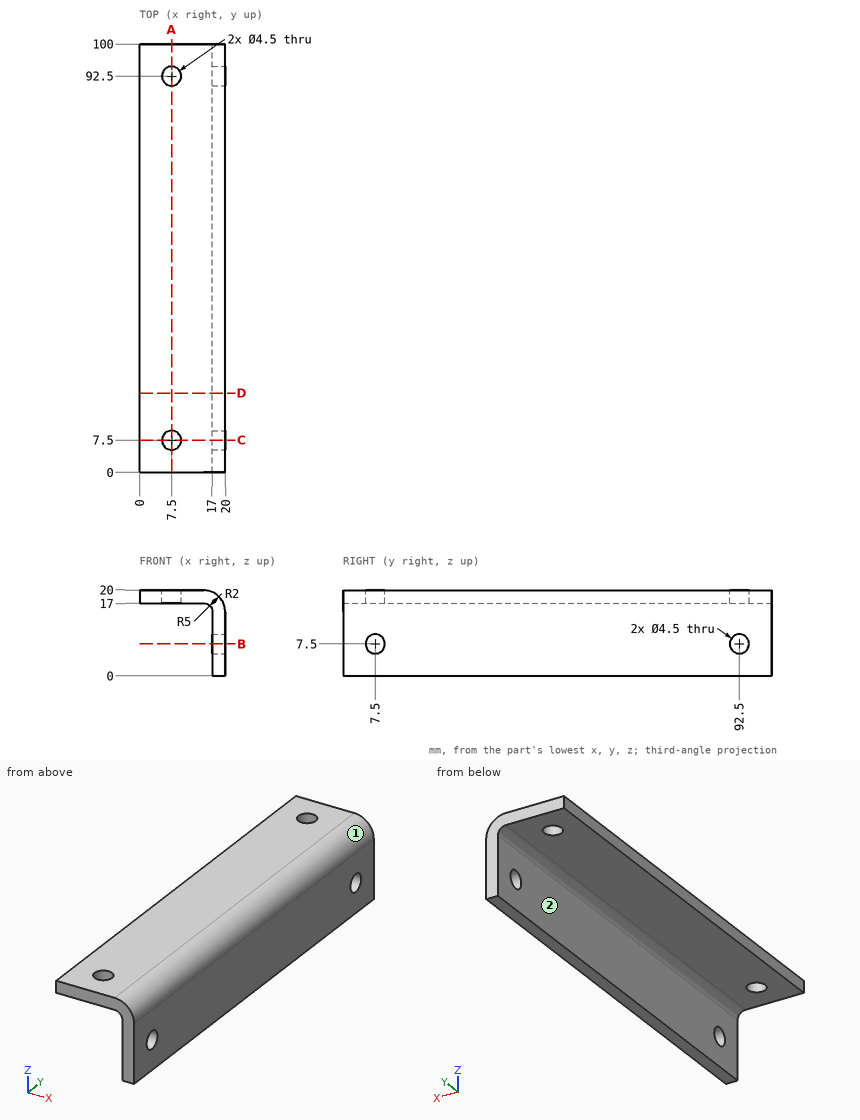
Verification items for this drawing (mm, ordinates from the low corner). A direction names the side the tool comes from. Coordinates: 2 decimals unless noted, no trailing zeros. Order: outer loops, then holes, each group sorted by start corner. A loop starts at its lowest first (then second) coordinate and runs counter-clockwise, first axis right, second up. Notation, with made-up numbers: M -1,75.5 L 13,75.5 A20 ccw 13,113.5 Z; hole C 31.5,21.5 d2. An arc over 180 degrees is marked long. One line per item, written item: value. Start each with the question number.
Item 1: Access from +Z, -Z, +X, -X, +Y, -Y to the whole of each face (thin tool, end or side, straight path). Record for the marked faces 1 and 2.
Item 2: Sectioned sample at C-C on y = 7.5. Record the cut outline in (x, z), then the cut area to 3 significant figures.
Item 3: Thickness scan on probe 1 along Y at (x, z) = (7.5, 19.2); probe 2 along Y at (x, z) = (9.5, 17.5); probe 3 along Z at (x, y) = (10.5, 57.5). Record the ranges inside material, lowest first.
Item 4: Depth check by flat-ended pin: P1, Ø7.5, axis at x = 8.5, y = 70.5, coming from the -Z side. Enter the tip coordinate at first touch or a pass-through.
Item 5: Sectioned sample at A-A on x = 7.5. Record the cut outline in (y, z).
Item 6: Sectioned sample at D-D on y = 18.5. Record the cut outline in (x, z).
Item 7: Sectioned sample at B-B on z = 7.5. Record the cut outline in (x, y), then the cut area to 3 significant figures.
Calculated:
1. face 1: +Z, +X, +Y, -Y
1. face 2: -Z, -X, +Y, -Y
2. outline: M 0,17 L 5.25,17 L 5.25,20 L 0,20 Z; M 9.75,17 L 15,17 A2 cw 17,15 L 17,9.75 L 20,9.75 L 20,15 A5 ccw 15,20 L 9.75,20 Z; M 17,0 L 20,0 L 20,5.25 L 17,5.25 Z
2. area: 79.5 mm^2
3. probe 1: 0 to 5.25, 9.75 to 90.25, 94.75 to 100
3. probe 2: 0 to 6.47, 8.53 to 91.47, 93.53 to 100
3. probe 3: 17 to 20
4. P1: z = 17
5. outline: M 0,17 L 5.25,17 L 5.25,20 L 0,20 Z; M 9.75,17 L 90.25,17 L 90.25,20 L 9.75,20 Z; M 94.75,17 L 100,17 L 100,20 L 94.75,20 Z
6. outline: M 0,17 L 15,17 A2 cw 17,15 L 17,0 L 20,0 L 20,15 A5 ccw 15,20 L 0,20 Z
7. outline: M 17,0 L 20,0 L 20,5.25 L 17,5.25 Z; M 17,9.75 L 20,9.75 L 20,90.25 L 17,90.25 Z; M 17,94.75 L 20,94.75 L 20,100 L 17,100 Z
7. area: 273 mm^2
